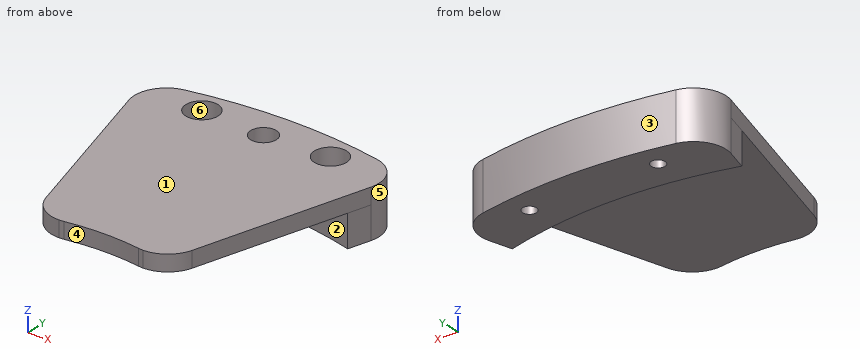
```python
from build123d import *

# Parameters (mm, degrees)
EXTRUDE_1_DEPTH     = 5
EXTRUDE_START       = 10
EXTRUDE_2_DEPTH     = 10
SKETCH_3_R          = 2.15
CUT_EXTRUDE_1_DEPTH = 50
SKETCH_4_R          = 5
CUT_EXTRUDE_2_DEPTH = 10


with BuildPart() as part:
    # 草图1 → 凸台-拉伸1 (new body)
    with BuildSketch(Plane.XY):
        with BuildLine():
            Line((-37.630075072, 134.476679949), (-22.746271228, 81.287189306))
            ThreePointArc((-22.746271228, 81.287189306), (-19.159893018, 76.014894835), (-13.116196156, 73.981934953))
            ThreePointArc((-13.116196156, 73.981934953), (-12.342334545, 74.011923006), (-11.573114255, 74.101707311))
            ThreePointArc((-11.573114255, 74.101707311), (0, 75), (11.573114255, 74.101707311))
            ThreePointArc((11.573114255, 74.101707311), (12.342334545, 74.011923006), (13.116196156, 73.981934953))
            ThreePointArc((13.116196156, 73.981934953), (19.159893018, 76.014894835), (22.746271228, 81.287189306))
            Line((22.746271228, 81.287189306), (37.630075072, 134.476679949))
            ThreePointArc((37.630075072, 134.476679949), (36.534141944, 142.38375917), (30, 146.969384567))
            ThreePointArc((30, 146.969384567), (0, 150), (-30, 146.969384567))
            ThreePointArc((-30, 146.969384567), (-36.534141944, 142.38375917), (-37.630075072, 134.476679949))
        make_face()
        with BuildLine():
            ThreePointArc((0, 144), (-4, 140), (0, 136))
            ThreePointArc((0, 136), (4, 140), (0, 144))
        make_face(mode=Mode.SUBTRACT)
    extrude(amount=EXTRUDE_1_DEPTH)

    # 草图2 → 凸台-拉伸2 (add)
    with BuildSketch(Plane(origin=(0, 0, 0), x_dir=(-1, 0, 0), z_dir=(0, 0, -1)).offset(EXTRUDE_START)):
        with BuildLine():
            Line((37.630075072, 134.476679949), (35.705379823, 127.598494708))
            ThreePointArc((35.705379823, 127.598494708), (0, 132.5), (-35.705379823, 127.598494708))
            Line((-35.705379823, 127.598494708), (-37.630075072, 134.476679949))
            ThreePointArc((-37.630075072, 134.476679949), (-36.534141944, 142.38375917), (-30, 146.969384567))
            ThreePointArc((-30, 146.969384567), (0, 150), (30, 146.969384567))
            ThreePointArc((30, 146.969384567), (36.534141944, 142.38375917), (37.630075072, 134.476679949))
        make_face()
    extrude(amount=-EXTRUDE_2_DEPTH)

    # 草图3 → 切除-拉伸1 (cut)
    with BuildSketch(Plane.XY.offset(5)):
        with Locations((-20, 141.089510595)):
            Circle(SKETCH_3_R)
        with Locations((20, 141.089510595)):
            Circle(SKETCH_3_R)
    extrude(amount=-CUT_EXTRUDE_1_DEPTH, mode=Mode.SUBTRACT)

    # 草图4 → 切除-拉伸2 (cut)
    with BuildSketch(Plane.XY.offset(5)):
        with Locations((-20, 141.089510595)):
            Circle(SKETCH_4_R)
        with Locations((20, 141.089510595)):
            Circle(SKETCH_4_R)
    extrude(amount=-CUT_EXTRUDE_2_DEPTH, mode=Mode.SUBTRACT)


solid = part.part
```
Input: part model. Units: mm. Frame: model coordinates. Face numbers are marked on the shaded views. A direction names the side the tool comes from. Give positions to 0.01 mm unless a question says otherwise; leave off trailing zeros. Write each loop counter-clockwise with the first axis right and the second up, starting at its lowest first coordinate (ties: lowest second). Pieces come first, ordered by that corner, then holes. Notation, with made-up numbers: (-33, -31.75) - (24, -31.75) arc R14 cw to (24, -24.75) - close; hole circle Ø10 at (86.5, 77). An arc over 180 degrees is marked (long way). Write item = value, one per line. Start each with the question number.
1. Section query A-A, the plane x = 0. Output: boundary loops of the cut face in (y, z).
2. Section query B-B, the plane z = 1.5. Output: boundary loops of the cut face in (x, y), then the cut area to 3 significant figures.
3. Section query D-D, the plane x = -20. Output: boundary loops of the cut face in (y, z), then the cut area to 3 significant figures.
4. Ray query, L1, parallel to Z at x = -3.5, y = 123.5; L2, parallel to Y at x = -20, z = 2.75; L3, parallel to Y at x = 20, z = -2.5. Return the intervals inside material, ascending.
5. Mould query, pull axis X, two halves, no side actions, for the marked faces 1, 2, 3 and 4. Classes: released by +X, released by -X, zero draft, split by the parting line, or undercut.
6. First-contact query: pin 1 Ø1.5 at (x, z) = (30.5, -0.5) entering from +Y; pin 2 Ø4 at (x, y) = (-20, 141.09) entering from -Z; pin 3 Ø1.5 at (x, z) = (4, -1) entering from +Y; pin 4 Ø4 at (x, z) = (11.5, -1.5) entering from -Y. Flat tips, straight axial feed; report the tip coordinate or a pass-through.
7. Section query C-C, the plane y = 140. Output: boundary loops of the cut face in (x, z).
8. Access query for the marked faces 5 and 6. Directions: +Z, -Z, +X, -X, +Y, -Y. A direction counts if a zero-diameter tool reaches every point of the face in a straight line with its end or side. Return the directions, or none.
Check sheet entries:
q1.outline = (75, 0) - (132.5, 0) - (132.5, -10) - (150, -10) - (150, 5) - (144, 5) - (144, 0) - (136, 0) - (136, 5) - (75, 5) - close
q2.outline = (-37.63, 134.48) - (-22.75, 81.29) arc R10 ccw to (-11.57, 74.1) arc R75 cw to (11.57, 74.1) arc R10 ccw to (22.75, 81.29) - (37.63, 134.48) arc R10 ccw to (30, 146.97) arc R150 ccw to (-30, 146.97) arc R10 ccw to start; hole circle Ø10 at (-20, 141.09); hole circle Ø8 at (0, 140); hole circle Ø10 at (20, 141.09)
q2.area = 4,310 mm2
q3.outline = (76.73, 0) - (130.98, 0) - (130.98, -10) - (138.94, -10) - (138.94, -5) - (136.09, -5) - (136.09, 5) - (76.73, 5) - close; (143.24, -10) - (148.66, -10) - (148.66, 5) - (146.09, 5) - (146.09, -5) - (143.24, -5) - close
q3.area = 415 mm2
q4.L1 = 0 to 5
q4.L2 = 76.73 to 136.09, 146.09 to 148.66
q4.L3 = 130.98 to 136.09, 146.09 to 148.66
q5.face_1 = zero draft
q5.face_2 = undercut
q5.face_3 = split by the parting line
q5.face_4 = undercut
q6.pin_1 = 147.02
q6.pin_2 = through
q6.pin_3 = 149.96
q6.pin_4 = 73.99
q7.outline = (-37.59, -10) - (-21.85, -10) - (-21.85, -5) - (-24.88, -5) - (-24.88, 5) - (-37.59, 5) - close; (-18.15, -10) - (18.15, -10) - (18.15, -5) - (15.12, -5) - (15.12, 5) - (4, 5) - (4, 0) - (-4, 0) - (-4, 5) - (-15.12, 5) - (-15.12, -5) - (-18.15, -5) - close; (21.85, -10) - (37.59, -10) - (37.59, 5) - (24.88, 5) - (24.88, -5) - (21.85, -5) - close
q8.face_5 = +Z, -Z, +X
q8.face_6 = +Z
